```python
from build123d import *

# Parameters (mm, degrees)
F0_W     = 15
F0_H     = 15
F1_DEPTH = 2
F3_D     = 2
F4_R     = 1


with BuildPart() as f1:
    # F0 (on Top) → F1 (new body)
    with BuildSketch(Plane.XY):
        with Locations((-7.5, 7.5)):
            Rectangle(F0_W, F0_H)
    extrude(amount=F1_DEPTH)

    # F3 (through all)
    with Locations(Plane.XY.offset(2)):
        with Locations((-7.5, 7.5)):
            Hole(F3_D / 2)

    # F4
    f4_edges = [f1.edges().sort_by_distance(p)[0] for p in [
        (-7.5, 0, 2),
        (-15, 7.5, 2),
        (-7.5, 15, 2),
        (0, 7.5, 2),
        (0, 0, 1),
        (-15, 0, 1),
        (0, 15, 1),
        (-15, 15, 1),
    ]]
    fillet(f4_edges, radius=F4_R)


solid = f1.part
```
Build history of the part. All positions in model axes, mm. Coordinates: 2 decimals unless noted, no trailing zeros. Order: outer loops, then holes, each group sorted by start corner. A loop starts at its lowest first (then second) coordinate and runs counter-clockwise, first axis right, second up. Notation, with made-up numbers: (73.25, 29) -> (110.25, 29) arc R12 ccw to (110.25, 43) -> close; hole circle Ø9 at (-12.75, -4). An arc over 180 degrees is marked (long way). Answer in a Markdown table with one row per item. Add a question column.
Q1. Band-saw the part on C-C, the plane z = 0.45. List the corners of the cut face in (x, y).
Q2. Wall check: line 1 along Y through (x, z) = (-7.5, 0.4); line 2 along Y through (x, z) = (-7.5, 1.6); line 3 along Y through (x, z) = (-2.25, 1.1). Give the ranges that are in metal, low to high. Write a range as [from, to].
Q3. Mould opens along Y. For faces 1 (the face through (-0.301, 14.715, 0.507)), 2 (the face through (-7.6, 0, 0.5)), 3 (the face through (-7.37, 8.49, 0.99)) say: +Y half, -Y half, draft (parallel to the pull), parting line (faces both ways), or undercut.
Q4. Band-saw the part on A-A, the plane x = -7.5. List the corners of the cut face in (y, z), then the cut area to 3 significant figures.
Q5. Band-saw the part on B-B, the plane y = 7.5. List the corners of the cut face in (x, z), then the cut area to 3 significant figures.
Q6. Band-saw the part on D-D, the plane z = 1.6. List the corners of the cut face in (x, y).
Answers follow:
| question | item | result |
|---|---|---|
| 1 | outline | (-15, 1) arc R1 ccw to (-14, 0) -> (-1, 0) arc R1 ccw to (0, 1) -> (0, 14) arc R1 ccw to (-1, 15) -> (-14, 15) arc R1 ccw to (-15, 14) -> close; hole circle Ø2 at (-7.5, 7.5) |
| 2 | line 1 | [0, 6.5], [8.5, 15] |
| 2 | line 2 | [0.2, 6.5], [8.5, 14.8] |
| 2 | line 3 | [0.01, 14.99] |
| 3 | face 1 | +Y half |
| 3 | face 2 | -Y half |
| 3 | face 3 | undercut |
| 4 | outline | (0, 0) -> (6.5, 0) -> (6.5, 2) -> (1, 2) arc R1 ccw to (0, 1) -> close; (8.5, 0) -> (15, 0) -> (15, 1) arc R1 ccw to (14, 2) -> (8.5, 2) -> close |
| 4 | area | 25.6 mm^2 |
| 5 | outline | (-15, 0) -> (-8.5, 0) -> (-8.5, 2) -> (-14, 2) arc R1 ccw to (-15, 1) -> close; (-6.5, 0) -> (0, 0) -> (0, 1) arc R1 ccw to (-1, 2) -> (-6.5, 2) -> close |
| 5 | area | 25.6 mm^2 |
| 6 | outline | (-14.8, 1) arc R0.8 ccw to (-14, 0.2) -> (-1, 0.2) arc R0.8 ccw to (-0.2, 1) -> (-0.2, 14) arc R0.8 ccw to (-1, 14.8) -> (-14, 14.8) arc R0.8 ccw to (-14.8, 14) -> close; hole circle Ø2 at (-7.5, 7.5) |
